Can you work these out from the model? Positions are in its coordinate system, mm. Round coordinates to 2 decimals unless told otherwise and drop trailing zeros. Write each loop counter-clockwise with the first axis right and the second up, starting at its lowest first coordinate (ties: lowest second). Pieces come first, ordered by that corner, then holes. Notation, with made-up numbers: M 34,24 L 50,24 A27 cw 50,63 Z; hole C -10.75,-33 d4. An arc over 180 degrees is marked long. Answer in a Markdown table with one row per item. Add a question column.
(1) Suppose I cut it at C-C, the plane x = 1. Write out the boundary of the cut face in (y, z), then the cut area to 3 significant figures.
(2) If we mould it in two halves opening along X, with no side actions, what happens to faces 1 (the face through (44, -35, 1.588)), 2 (the face through (57.488, -14.967, 0.783)), 3 (the face through (99.77, -33.24, 0.78)), 4 (the face through (89.238, -21.317, 0.783))? For each: released by +X, released by -X, zero draft, split by the parting line, or undercut.
(3) Suppose I cut it at A-A, the plane z = 0.6. Write out the boundary of the cut face in (x, y), then the cut area to 3 significant figures.
(4) If I drill on probe 1 along X at (y, z) = (-19.5, 1.35); probe 2 along X at (y, z) = (-14, 1); probe 3 along X at (y, z) = (-37, 0.8), over which ranges is the centre line in solid material (lowest first)?
(5) I'm going to push a flat-ended pin straight in: pin 1 (3.5 mm diameter, centred on x = 91.47, y = -21.22, fed in from -Z). Where does the tip first touch, or does it pass through?
(6) Suppose I cut it at B-B, the plane y = -34.5. Write out the boundary of the cut face in (x, z), then the cut area to 3 significant figures.
Autodesk Inventor part; units mm, degrees
ref_plane "YZ Plane" through (0, 0, 0) normal (1, 0, 0) x (0, 1, 0)
ref_plane "XZ Plane" through (0, 0, 0) normal (0, 1, 0) x (-1, 0, 0)
ref_plane "XY Plane" through (0, 0, 0) normal (0, 0, 1) x (1, 0, 0)
sketch "Sketch1" plane through (0, 0, 0) normal (0, 0, 1) x (1, 0, 0)
  circle A0 centre (53.3707, -52.9691) radius 2.2352
  arc A1 (-7.0885, -40.7359) -> (4.0322, -62.6709) centre (2.7723, -49.5231) ccw
  arc A2 (94.5267, -13.6218) -> (87.3345, -8.5191) centre (87.3345, -16.1391) ccw
  line L0 (25.0369, -8.5191) -> (87.3345, -8.5191)
  arc A3 (96.8127, -37.2153) -> (99.7022, -28.4091) centre (92.51, -30.9263) ccw
  line L1 (99.7022, -28.4091) -> (94.5267, -13.6218)
  arc A4 (59.2846, -57.3763) -> (76.4278, -51.1618) centre (55.7999, -21.0109) ccw
  arc A5 (25.0369, -8.5191) -> (19.348, -11.0695) centre (25.0369, -16.1391) ccw
  circle A6 centre (59.7207, -27.5691) radius 2.2352
  circle A7 centre (91.4707, -21.2191) radius 2.2352
  circle A8 centre (59.7207, -14.8691) radius 2.2352
  line L2 (76.4278, -51.1618) -> (96.8127, -37.2153)
  line L3 (19.348, -11.0695) -> (-7.0885, -40.7359)
  line L4 (4.0322, -62.6709) -> (59.2846, -57.3763)
  point P0 (0, 0)
  point P1 (19.348, -11.0695)
  point P2 (-7.0885, -40.7359)
  point P3 (4.0322, -62.6709)
  point P4 (59.2846, -57.3763)
  point P5 (76.4278, -51.1618)
  point P6 (94.5267, -13.6218)
  point P7 (87.3345, -8.5191)
extrude "Extrusion1" add sketch "Sketch1" along normal blind 1.5875
properties part number "neil"
Calculated:
| question | item | result |
|---|---|---|
| 1 | outline | M -62.61,0 L -31.66,0 L -31.66,1.59 L -62.61,1.59 Z |
| 1 | area | 49.1 mm² |
| 2 | face 1 | zero draft |
| 2 | face 2 | undercut |
| 2 | face 3 | released by +X |
| 2 | face 4 | undercut |
| 3 | outline | M -7.09,-40.74 A13.21 ccw 4.03,-62.67 L 59.28,-57.38 A36.53 ccw 76.43,-51.16 L 96.81,-37.22 A7.62 ccw 99.7,-28.41 L 94.53,-13.62 A7.62 ccw 87.33,-8.52 L 25.04,-8.52 A7.62 ccw 19.35,-11.07 Z; hole C 53.37,-52.97 d4.47; hole C 59.72,-27.57 d4.47; hole C 59.72,-14.87 d4.47; hole C 91.47,-21.22 d4.47 |
| 3 | area | 4,480 mm² |
| 4 | probe 1 | 11.84 to 90.04, 92.9 to 96.58 |
| 4 | probe 2 | 16.74 to 57.66, 61.78 to 94.66 |
| 4 | probe 3 | -3.76 to 97.11 |
| 5 | pin 1 | through |
| 6 | outline | M -1.53,0 L 99.24,0 L 99.24,1.59 L -1.53,1.59 Z |
| 6 | area | 160 mm² |
